Build history of the part. All positions in model axes, mm. A direction names the side the tool comes from. Give positions to 0.01 mm unless a question says otherwise; leave off trailing zeros. Loops run counter-clockwise (first coordinate to the right, second up) from the corner with the lowest first, then second, coordinate; pieces in that order, holes last.
1) Wall check: line 1 (Y direction, x = 75, z = 4.1); line 2 (Z direction, x = -39, y = -57.5); line 3 (X direction, y = 50, z = 3.45). Give the ranges that are in metal, low to high.
2) Band-saw the part on A-A on z = 4.2. List the corners of the cut face in (x, y).
3) 3-axis set-ups, long thin cutter, end or side, ignore diameter. For faces 3 (the cylindrical face through (-83.825, 49.545, 4.479)), 4 (the cylindrical face through (-81.3, -101.3, 3)): which of +Z, -Z, +X, -X, +Y, -Y reach the whole face in a straight line?
4) Two-plate mould, pull along Y, no slides. Class faces 1 (the cylindrical face through (78.262, 28.057, 2.958)), 2 (the flat face through (-79.5, 50.2, 6)): +Y half, -Y half, draft (parallel to the pull), parting line (faces both ways), or undercut.
5) Flat gauge pins, fed straight in: P1, Ø8, axis at x = -45, y = -79, coming from the +Z side; P2, Ø6.5, axis at x = 76.43, y = -103.27, coming from the +Z side. Where does each tip first touch, or does it go through?
6) Band-saw the part on C-C on x = -32. List the corners of the cut face in (y, z).
7) Band-saw the part on B-B on y = -27.5. List the corners of the cut face in (x, z).
```python
from build123d import *

# Parameters (mm, degrees)
F0_W     = 170.19
F0_H     = 170.18
F0_R     = 3.5
F1_DEPTH = 3
F0_R_2   = 1.98
F2_DEPTH = 6


with BuildPart() as f1:
    # F0 (on Top) → F1 (new body)
    with BuildSketch(Plane.XY):
        with Locations((-2.9422, -23.25511)):
            Rectangle(F0_W, F0_H)
        with Locations((-81.0472, -103.26511)):
            Circle(F0_R, mode=Mode.SUBTRACT)
        with Locations((76.4328, -103.26511)):
            Circle(F0_R, mode=Mode.SUBTRACT)
        with Locations((-81.0472, 51.67489)):
            Circle(F0_R, mode=Mode.SUBTRACT)
        with Locations((76.4328, 28.81489)):
            Circle(F0_R, mode=Mode.SUBTRACT)
    extrude(amount=F1_DEPTH)

    # F0 (on Top) → F2 (join)
    with BuildSketch(Plane.XY):
        with Locations((76.4328, -103.26511)):
            Circle(F0_R)
        with Locations((76.4328, -103.26511)):
            Circle(F0_R_2, mode=Mode.SUBTRACT)
        with Locations((-81.0472, -103.26511)):
            Circle(F0_R)
        with Locations((-81.0472, -103.26511)):
            Circle(F0_R_2, mode=Mode.SUBTRACT)
        with Locations((-81.0472, 51.67489)):
            Circle(F0_R)
        with Locations((-81.0472, 51.67489)):
            Circle(F0_R_2, mode=Mode.SUBTRACT)
        with Locations((76.4328, 28.81489)):
            Circle(F0_R)
        with Locations((76.4328, 28.81489)):
            Circle(F0_R_2, mode=Mode.SUBTRACT)
    extrude(amount=F2_DEPTH)


solid = f1.part
```
Findings below:
1. line 1: y = -106.46 to -104.63, -101.9 to -100.07, 25.62 to 27.45, 30.18 to 32.01
1. line 2: z = 0 to 3
1. line 3: x = -84.12 to -82.1, -79.99 to -77.97
2. outline: circle Ø7 at (-81.05, -103.27); circle Ø7 at (-81.05, 51.67); circle Ø7 at (76.43, -103.27); circle Ø7 at (76.43, 28.81); hole circle Ø3.96 at (-81.05, -103.27); hole circle Ø3.96 at (-81.05, 51.67); hole circle Ø3.96 at (76.43, -103.27); hole circle Ø3.96 at (76.43, 28.81)
3. face 3: +Z
3. face 4: +Z, -Z
4. face 1: undercut
4. face 2: draft
5. P1: stops at z = 3
5. P2: stops at z = 6
6. outline: (-108.35, 0) - (61.83, 0) - (61.83, 3) - (-108.35, 3) - close
7. outline: (-88.04, 0) - (82.15, 0) - (82.15, 3) - (-88.04, 3) - close
